The model under review builds one solid part; all positions refer to its coordinate system, in mm. Face numbers are marked on the shaded views. A direction names the side the tool comes from. Give positions to 0.01 mm unless a question says otherwise; leave off trailing zeros. Loops run counter-clockwise (first coordinate to the right, second up) from the corner with the lowest first, then second, coordinate; pieces in that order, holes last. Notation, with made-up numbers: (68, 28.25) -> (107, 28.25) arc R17 cw to (107, 38.25) -> close; hole circle Ø11 at (21, -1.5). An arc over 180 degrees is marked (long way). Write each question's results on one line, items separated by ' | '. Start each with the question number.
Q1. Wall thickness on L1, parallel to Y at x = 1.5, z = 15.5; L2, parallel to Z at x = -3, y = -2; L3, parallel to Z at x = -1, y = -4.75: over which ranges is each line inside the solid? List them lowest first. Write a range as [from, to].
Q2. We need section D-D (x = -4.75). Write out the cut boundary in (y, z), plus the area to 3 significant figures.
Q3. We need section C-C (z = 14). Write out the cut boundary in (x, y).
Q4. Insertion check: pin 1 Ø5 at (x, y) = (2.5, -5.5) entering from -Z; pin 2 Ø1.6 at (y, z) = (0, 16.5) entering from -X; pin 3 Ø1.5 at (y, z) = (-0.5, 13) entering from -X. Each pin has a flat end and moves straight along its axis. Give the tip position at first contact, or say it passes through.
Q5. Machinability: for the marked faces 1, 2 and 3, which of the approach directions +Z, -Z, +X, -X, +Y, -Y give a long, thin tool a straight path to every point of the face, cutting with its end or side? Answer none if there is none.
Q6. We need section B-B (y = 0). Write out the cut boundary in (x, z), plus the area to 3 significant figures.
Q7. We need section A-A (x = 0). Write out the cut boundary in (y, z).
Autodesk Inventor part; units mm, degrees
ref_plane "YZ Plane" through (0, 0, 0) normal (1, 0, 0) x (0, 1, 0)
ref_plane "XZ Plane" through (0, 0, 0) normal (0, 1, 0) x (-1, 0, 0)
ref_plane "XY Plane" through (0, 0, 0) normal (0, 0, 1) x (1, 0, 0)
sketch "Sketch1" plane through (0, 0, 0) normal (0, 0, 1) x (1, 0, 0)
  line L0 (-6, 6.5) -> (6, 6.5)
  line L1 (6, 6.5) -> (6, -6.5)
  line L2 (6, -6.5) -> (-6, -6.5)
  line L3 (-6, -6.5) -> (-6, 6.5)
  line L4 (-6, 6.5) -> (6, -6.5) construction
  line L5 (6, 6.5) -> (-6, -6.5) construction
  point P0 (0, 0)
  dimension "d0" = 12
  dimension "d1" = 13
extrude "Extrusion1" add sketch "Sketch1" along normal blind 9
sketch "Sketch2" plane through (0, 0, 9) normal (0, 0, 1) x (1, 0, 0)
  line L0 (-6, -6.5) -> (6, -6.5)
  line L1 (6, -6.5) -> (6, 6.5)
  line L2 (6, 6.5) -> (-6, 6.5)
  line L3 (-6, 6.5) -> (-6, -6.5)
  line L4 (6, 6.5) -> (-6, 6.5)
  line L5 (-6, 6.5) -> (-3, 6.5)
  line L6 (-3, 6.5) -> (-3, 7)
  line L7 (-3, 7) -> (-6, 7)
  line L8 (-6, 7) -> (-6, 6.5)
  line L9 (6, 6.5) -> (3, 6.5)
  line L10 (3, 6.5) -> (3, 7)
  line L11 (3, 7) -> (6, 7)
  line L12 (6, 7) -> (6, 6.5)
  line L13 (-6, -6.5) -> (6, -6.5)
  line L14 (6, -6.5) -> (3, -6.5)
  line L15 (3, -6.5) -> (3, -7)
  line L16 (3, -7) -> (6, -7)
  line L17 (6, -7) -> (6, -6.5)
  line L18 (-6, -6.5) -> (-3, -6.5)
  line L19 (-3, -6.5) -> (-3, -7)
  line L20 (-3, -7) -> (-6, -7)
  line L21 (-6, -7) -> (-6, -6.5)
  point P0 (0, 0)
  dimension "d4" = 3
  dimension "d5" = 0.5
extrude "Extrusion2" add sketch "Sketch2" along normal blind 1.5
sketch "Sketch3" plane through (0, 0, 10.5) normal (0, 0, 1) x (1, 0, 0)
  circle A0 centre (0, 0) radius 4
  dimension "d8" = 8
extrude "Extrusion3" add sketch "Sketch3" along normal blind 3
sketch "Sketch4" plane through (0, 0, 13.5) normal (0, 0, 1) x (1, 0, 0)
  line L0 (-3, 0.75) -> (3, 0.75)
  line L1 (3, 0.75) -> (3, -0.75)
  line L2 (3, -0.75) -> (-3, -0.75)
  line L3 (-3, -0.75) -> (-3, 0.75)
  line L4 (-3, 0.75) -> (3, -0.75) construction
  line L5 (3, 0.75) -> (-3, -0.75) construction
  point P0 (0, 0)
  dimension "d11" = 6
  dimension "d12" = 1.5
extrude "Extrusion4" add sketch "Sketch4" along normal blind 6
sketch "Sketch5" plane through (0, 0, 0) normal (0, 0, -1) x (-1, 0, 0)
  circle A0 centre (-1.9, 0) radius 0.5
  circle A1 centre (1.9, 0) radius 0.5
  point P0 (0, 0)
  dimension "d15" = 1
  dimension "d16" = 1
  dimension "d17" = 1.9
  dimension "d18" = 1.9
  dimension "d19" = 3.8
extrude "Extrusion5" add sketch "Sketch5" along normal blind 4.3
fillet "Fillet1" radius 0.2 2 edges at (2.4, 0, -4.3) (-1.4, 0, -4.3)
properties part number "KeyboardSwitch" material "ABS Plastic"
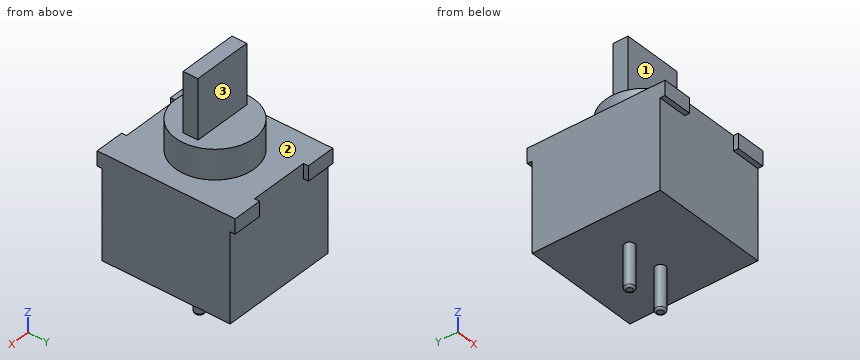
Output:
1) L1: [-0.75, 0.75] | L2: [0, 13.5] | L3: [0, 10.5]
2) outline: (-7, 9) -> (-6.5, 9) -> (-6.5, 0) -> (6.5, 0) -> (6.5, 9) -> (7, 9) -> (7, 10.5) -> (-7, 10.5) -> close | area: 138 mm2
3) outline: (-3, -0.75) -> (3, -0.75) -> (3, 0.75) -> (-3, 0.75) -> close
4) pin 1: z = 0 | pin 2: x = -3 | pin 3: x = -4
5) face 1: +Z, +X, -X, -Y | face 2: +Z | face 3: +Z, +X, -X, +Y
6) outline: (-6, 0) -> (-2.4, 0) -> (-2.4, -4.1) arc R0.2 ccw to (-2.2, -4.3) -> (-1.6, -4.3) arc R0.2 ccw to (-1.4, -4.1) -> (-1.4, 0) -> (1.4, 0) -> (1.4, -4.1) arc R0.2 ccw to (1.6, -4.3) -> (2.2, -4.3) arc R0.2 ccw to (2.4, -4.1) -> (2.4, 0) -> (6, 0) -> (6, 10.5) -> (4, 10.5) -> (4, 13.5) -> (3, 13.5) -> (3, 19.5) -> (-3, 19.5) -> (-3, 13.5) -> (-4, 13.5) -> (-4, 10.5) -> (-6, 10.5) -> close | area: 195 mm2
7) outline: (-6.5, 0) -> (6.5, 0) -> (6.5, 10.5) -> (4, 10.5) -> (4, 13.5) -> (0.75, 13.5) -> (0.75, 19.5) -> (-0.75, 19.5) -> (-0.75, 13.5) -> (-4, 13.5) -> (-4, 10.5) -> (-6.5, 10.5) -> close
